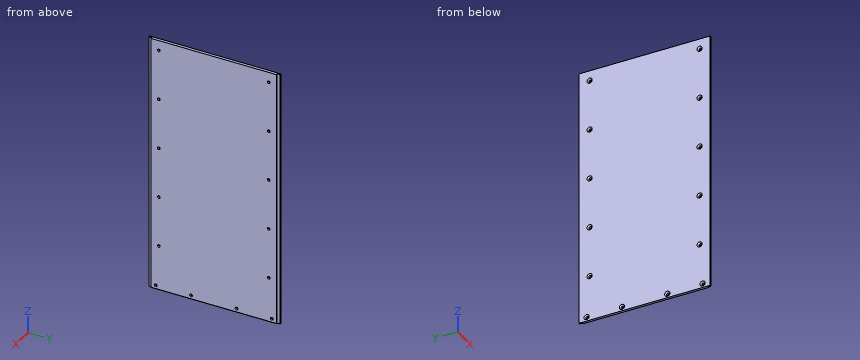
```python
from build123d import *

# Parameters (mm, degrees)
SKETCH1_W                                            = 510
SKETCH1_H                                            = 260
BOSS_EXTRUDE1_DEPTH                                  = 6
SKIZZE2_W                                            = 3
SKIZZE2_H                                            = 6
SCHNITT_LINEAR_AUSTRAGEN1_DEPTH                      = 527.34209408
FORMSENKUNG_FUR_M5_LINSENSENKSCHRAUBE_MI_D           = 5.5
FORMSENKUNG_FUR_M5_LINSENSENKSCHRAUBE_MI_CSINK_D     = 10.4
FORMSENKUNG_FUR_M5_LINSENSENKSCHRAUBE_MI_CSINK_ANGLE = 90
CHAMFER1_SIZE                                        = 1
CSK_FOR_M5_COUNTERSUNK_RAISED_HEAD_SCREW_D           = 5.5
CSK_FOR_M5_COUNTERSUNK_RAISED_HEAD_SCREW_CSINK_D     = 10.4
CSK_FOR_M5_COUNTERSUNK_RAISED_HEAD_SCREW_CSINK_ANGLE = 90
LPATTERN1_COUNT                                      = 5
LPATTERN1_PITCH                                      = 100
MIRROR1_COPY_1_D                                     = 5.5
MIRROR1_COPY_1_CSINK_D                               = 10.4
MIRROR1_COPY_1_CSINK_ANGLE                           = 90
MIRROR1_COPY_2_D                                     = 5.5
MIRROR1_COPY_2_CSINK_D                               = 10.4
MIRROR1_COPY_2_CSINK_ANGLE                           = 90
MIRROR1_COPY_3_D                                     = 5.5
MIRROR1_COPY_3_CSINK_D                               = 10.4
MIRROR1_COPY_3_CSINK_ANGLE                           = 90
MIRROR1_COPY_4_D                                     = 5.5
MIRROR1_COPY_4_CSINK_D                               = 10.4
MIRROR1_COPY_4_CSINK_ANGLE                           = 90


with BuildPart() as part:
    # Sketch1 → Boss-Extrude1 (new body)
    with BuildSketch(Plane(origin=(0, 0, 0), x_dir=(0, 0, -1), z_dir=(1, 0, 0))):
        Rectangle(SKETCH1_W, SKETCH1_H)
    extrude(amount=BOSS_EXTRUDE1_DEPTH)

    # Skizze2 → Schnitt-Linear austragen1 (cut, through all)
    with BuildSketch(Plane.XY.offset(255)):
        with Locations((4.5, 127)):
            Rectangle(SKIZZE2_W, SKIZZE2_H)
        with Locations((4.5, -127)):
            Rectangle(SKIZZE2_W, SKIZZE2_H)
    extrude(amount=-SCHNITT_LINEAR_AUSTRAGEN1_DEPTH, mode=Mode.SUBTRACT)

    # Formsenkung fur M5 Linsensenkschraube mit Schlitz1 (through all)
    with Locations(Plane.ZY):
        with Locations((-247, 115), (-247, 45)):
            formsenkung_fur_m5_linsensenkschraube_mi = CounterSinkHole(FORMSENKUNG_FUR_M5_LINSENSENKSCHRAUBE_MI_D / 2, FORMSENKUNG_FUR_M5_LINSENSENKSCHRAUBE_MI_CSINK_D / 2, counter_sink_angle=FORMSENKUNG_FUR_M5_LINSENSENKSCHRAUBE_MI_CSINK_ANGLE)

    # Spiegeln1: Formsenkung fur M5 Linsensenkschraube mit Schlitz1 across plane
    add(formsenkung_fur_m5_linsensenkschraube_mi.mirror(Plane.ZX), mode=Mode.SUBTRACT)

    # Chamfer1
    chamfer1_edges = [part.edges().sort_by_distance(p)[0] for p in [
        (6, 0, -255),
    ]]
    chamfer(chamfer1_edges, length=CHAMFER1_SIZE)

    # CSK for M5 Countersunk Raised Head Screw1 (through all)
    with Locations(Plane.ZY):
        with Locations((235, -109)):
            csk_for_m5_countersunk_raised_head_screw = CounterSinkHole(CSK_FOR_M5_COUNTERSUNK_RAISED_HEAD_SCREW_D / 2, CSK_FOR_M5_COUNTERSUNK_RAISED_HEAD_SCREW_CSINK_D / 2, counter_sink_angle=CSK_FOR_M5_COUNTERSUNK_RAISED_HEAD_SCREW_CSINK_ANGLE)

    # LPattern1: CSK for M5 Countersunk Raised Head Screw1 ×5
    with Locations(*[(0, 0, -i * LPATTERN1_PITCH) for i in range(1, LPATTERN1_COUNT)]):
        add(csk_for_m5_countersunk_raised_head_screw, mode=Mode.SUBTRACT)

    # Mirror1: CSK for M5 Countersunk Raised Head Screw1 across plane
    add(csk_for_m5_countersunk_raised_head_screw.mirror(Plane.ZX), mode=Mode.SUBTRACT)

    # Mirror1 copy 1 (through all)
    with Locations(Plane(origin=(0, 0, -100), x_dir=(0, 0, 1), z_dir=(-1, 0, 0))):
        with Locations((235, 109)):
            CounterSinkHole(MIRROR1_COPY_1_D / 2, MIRROR1_COPY_1_CSINK_D / 2, counter_sink_angle=MIRROR1_COPY_1_CSINK_ANGLE)

    # Mirror1 copy 2 (through all)
    with Locations(Plane(origin=(0, 0, -200), x_dir=(0, 0, 1), z_dir=(-1, 0, 0))):
        with Locations((235, 109)):
            CounterSinkHole(MIRROR1_COPY_2_D / 2, MIRROR1_COPY_2_CSINK_D / 2, counter_sink_angle=MIRROR1_COPY_2_CSINK_ANGLE)

    # Mirror1 copy 3 (through all)
    with Locations(Plane(origin=(0, 0, -300), x_dir=(0, 0, 1), z_dir=(-1, 0, 0))):
        with Locations((235, 109)):
            CounterSinkHole(MIRROR1_COPY_3_D / 2, MIRROR1_COPY_3_CSINK_D / 2, counter_sink_angle=MIRROR1_COPY_3_CSINK_ANGLE)

    # Mirror1 copy 4 (through all)
    with Locations(Plane(origin=(0, 0, -400), x_dir=(0, 0, 1), z_dir=(-1, 0, 0))):
        with Locations((235, 109)):
            CounterSinkHole(MIRROR1_COPY_4_D / 2, MIRROR1_COPY_4_CSINK_D / 2, counter_sink_angle=MIRROR1_COPY_4_CSINK_ANGLE)


solid = part.part
```
For this review, take the finished solid that the model builds, in its own axes (mm). Coordinates: 2 decimals unless noted, no trailing zeros. Write each loop counter-clockwise with the first axis right and the second up, starting at its lowest first coordinate (ties: lowest second). Pieces come first, ordered by that corner, then holes. Notation, with made-up numbers: (44, 18) - (89, 18) arc R17 ccw to (89, 48) - close; hole circle Ø8 at (13, 39.5). An arc over 180 degrees is marked (long way). Answer in a Markdown table with one row per item. Add a question column.
Q1. For probe 1 along Y at (x, z) = (3.3, 235); probe 2 along Z at (x, y) = (2.6, -115.5); probe 3 along Y at (x, z) = (5.65, 83), list the stretches that pass through material, from the lowest coordinate up.
Q2. For P1, Ø5, axis at y = -109, z = 235, coming from the -X side; P2, Ø9, axis at y = 109, z = 235, coming from the -X side; P3, Ø1.5, axis at x = 4.5, z = -5.5, coming from the +Y side; P4, Ø6.5, axis at y = 115, z = -247, coming from the -X side, all flat-tipped, find the tip position at first contact; note any pin that passes through.
Q3. We need section A-A, the plane z = 121.5. State the section outline as (x, y) points.
Answer list:
| question | item | result |
|---|---|---|
| 1 | probe 1 | y = -124 to -111.75, -106.25 to 106.25, 111.75 to 124 |
| 1 | probe 2 | z = -255 to -249.7, -244.3 to 255 |
| 1 | probe 3 | y = -124 to 124 |
| 2 | P1 | passes through |
| 2 | P2 | stops at x = 0.7 |
| 2 | P3 | stops at y = 124 |
| 2 | P4 | stops at x = 1.95 |
| 3 | outline | (0, -130) - (3, -130) - (3, -124) - (6, -124) - (6, 124) - (3, 124) - (3, 130) - (0, 130) - close |
